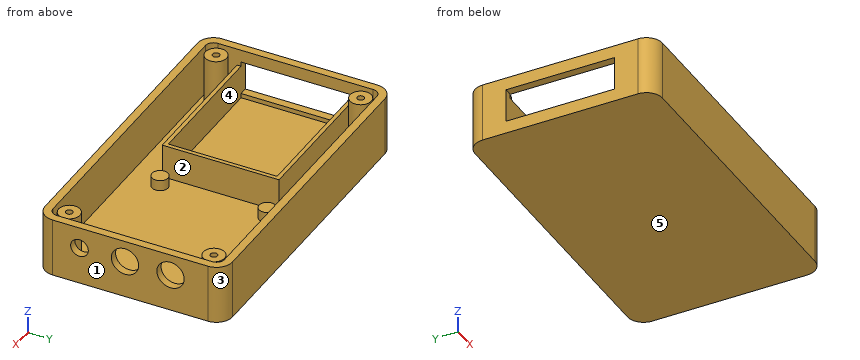
```python
from build123d import *

# Parameters (mm, degrees)
SKETCH1_W           = 120
SKETCH1_H           = 70
BOSS_EXTRUDE1_DEPTH = 22
FILLET1_R           = 6
SHELL1_T            = -3
SKETCH2_R           = 4
BOSS_EXTRUDE2_DEPTH = 18.0000001
SKETCH4_R           = 1.3
CUT_EXTRUDE1_DEPTH  = 4
BOSS_EXTRUDE3_DEPTH = 12.6
CUT_EXTRUDE2_REACH  = 128.921
SKETCH6_W           = 12.6
SKETCH6_H           = 40.6
CUT_EXTRUDE3_REACH  = 128.921
SKETCH8_R           = 5.1
SKETCH8_R_2         = 3.3
SKETCH9_R           = 3
BOSS_EXTRUDE4_DEPTH = 4


with BuildPart() as part:
    # Sketch1 → Boss-Extrude1 (new body)
    with BuildSketch(Plane.XY):
        Rectangle(SKETCH1_W, SKETCH1_H)
    extrude(amount=BOSS_EXTRUDE1_DEPTH)

    # Fillet1
    fillet1_edges = [part.edges().sort_by_distance(p)[0] for p in [
        (-60, 35, 11),
        (60, 35, 11),
        (60, -35, 11),
        (-60, -35, 11),
    ]]
    fillet(fillet1_edges, radius=FILLET1_R)

    # Shell1
    shell1_openings = [part.faces().sort_by_distance(p)[0] for p in [
        (0, 0, 22),
    ]]
    offset(amount=SHELL1_T, openings=shell1_openings, kind=Kind.INTERSECTION)

    # Sketch2 → Boss-Extrude2 (add)
    with BuildSketch(Plane.XY.offset(3)):
        with Locations((-52, -27)):
            Circle(SKETCH2_R)
        with Locations(Location((52, -27, 0), (0, 0, 180))):
            Circle(SKETCH2_R)
        with Locations((52, 27)):
            Circle(SKETCH2_R)
        with Locations(Location((-52, 27, 0), (0, 0, 180))):
            Circle(SKETCH2_R)
    extrude(amount=BOSS_EXTRUDE2_DEPTH)

    # Sketch4 → Cut-Extrude1 (cut)
    with BuildSketch(Plane.XY.offset(21.0000001)):
        with Locations((-52, 27)):
            Circle(SKETCH4_R)
        with Locations(Location((-52, -27, 0), (0, 0, 180))):
            Circle(SKETCH4_R)
        with Locations((52, -27)):
            Circle(SKETCH4_R)
        with Locations(Location((52, 27, 0), (0, 0, 180))):
            Circle(SKETCH4_R)
    extrude(amount=-CUT_EXTRUDE1_DEPTH, mode=Mode.SUBTRACT)

    # Sketch5 → Boss-Extrude3 (add)
    with BuildSketch(Plane(origin=(0, 0, 3), x_dir=(-1, 0, 0), z_dir=(0, 0, -1))):
        Polygon((57, 21.8), (4, 21.8), (4, -21.8), (57, -21.8), (57, -20.3), (5.5, -20.3), (5.5, 20.3), (57, 20.3), align=None)
    extrude(amount=-BOSS_EXTRUDE3_DEPTH)

    # Sketch6 → Cut-Extrude2 (cut, up to next)
    with BuildSketch(Plane(origin=(-60, 0, 0), x_dir=(0, 0, -1), z_dir=(1, 0, 0)), mode=Mode.PRIVATE) as cut_extrude2_sk1:
        with Locations((-11, 0)):
            Rectangle(SKETCH6_W, SKETCH6_H)
    cut_extrude2_tool1 = extrude(cut_extrude2_sk1.sketch, amount=CUT_EXTRUDE2_REACH, mode=Mode.PRIVATE) & part.part
    add(cut_extrude2_tool1.solids().sort_by_distance((-60, 0, 11))[0], mode=Mode.SUBTRACT)

    # Sketch8 → Cut-Extrude3 (cut, up to next)
    with BuildSketch(Plane.ZY.offset(-60), mode=Mode.PRIVATE) as cut_extrude3_sk1:
        with Locations(Location((14, 15, 0), (0, 0, 270))):
            Circle(SKETCH8_R)
    cut_extrude3_tool1 = extrude(cut_extrude3_sk1.sketch, amount=CUT_EXTRUDE3_REACH, mode=Mode.PRIVATE) & part.part
    # Sketch8 → Cut-Extrude3 (cut, up to next)
    with BuildSketch(Plane.ZY.offset(-60), mode=Mode.PRIVATE) as cut_extrude3_sk2:
        with Locations(Location((14, -2, 0), (0, 0, 270))):
            Circle(SKETCH8_R)
    cut_extrude3_tool2 = extrude(cut_extrude3_sk2.sketch, amount=CUT_EXTRUDE3_REACH, mode=Mode.PRIVATE) & part.part
    # Sketch8 → Cut-Extrude3 (cut, up to next)
    with BuildSketch(Plane.ZY.offset(-60), mode=Mode.PRIVATE) as cut_extrude3_sk3:
        with Locations(Location((14, -19, 0), (0, 0, 270))):
            Circle(SKETCH8_R_2)
    cut_extrude3_tool3 = extrude(cut_extrude3_sk3.sketch, amount=CUT_EXTRUDE3_REACH, mode=Mode.PRIVATE) & part.part
    add(cut_extrude3_tool1.solids().sort_by_distance((60, 15, 14))[0], mode=Mode.SUBTRACT)
    add(cut_extrude3_tool2.solids().sort_by_distance((60, -2, 14))[0], mode=Mode.SUBTRACT)
    add(cut_extrude3_tool3.solids().sort_by_distance((60, -19, 14))[0], mode=Mode.SUBTRACT)

    # Sketch9 → Boss-Extrude4 (add)
    with BuildSketch(Plane.XY.offset(3)):
        with Locations((43, 20)):
            Circle(SKETCH9_R)
        with Locations((1, 20)):
            Circle(SKETCH9_R)
        with Locations(Location((1, -20, 0), (0, 0, 180))):
            Circle(SKETCH9_R)
        with Locations(Location((43, -20, 0), (0, 0, 180))):
            Circle(SKETCH9_R)
    extrude(amount=BOSS_EXTRUDE4_DEPTH)


solid = part.part
```
Work out the finished part from the listing and answer in its coordinate system (mm). Face numbers are marked on the shaded views. A direction names the side the tool comes from. Round coordinates to 2 decimals unless told otherwise and drop trailing zeros. Write each loop counter-clockwise with the first axis right and the second up, starting at its lowest first coordinate (ties: lowest second). Pieces come first, ordered by that corner, then holes.
1) A cutting plane is placed at A-A on y = 15. Determine the outline of the cut face in (x, z), and give its area (4 significant figures).
2) Determine the mould class of the marked faces 3, 4 and 5 for opening direction Y: pulls with the +Y half, pulls with the -Y half, needs draft (parallel to the pull), parting line crosses it, or undercut.
3) A cutting plane is placed at D-D on x = -38.5. Determine the outline of the cut face in (y, z), and give its area (3 significant figures).
4) Flat-ended cylindrical pins translate along their axes: P1, Ø4, axis at y = -1, z = 8.5, coming from the -X side; P2, Ø2.5, axis at x = 52.5, y = 26.5, coming from the +Z side; P3, Ø1, axis at x = -23, y = -8, coming from the +Z side. Find the tip coordinate at first contact, or state that the pin passes through.
5) A cutting plane is placed at B-B on x = 1. Determine the outline of the cut face in (y, z), and give its area (3 significant figures).
6) A cutting plane is placed at C-C on y = 27. Determine the outline of the cut face in (x, z).
7) Which of the six approach directions +Z, -Z, +X, -X, +Y, -Y give full straight-line access (tool end or side, diameter ignored) to the marked faces 1 and 2?
8) Consider probe 1 along Y at (x, z) = (52, 18); probe 2 along Y at (x, z) = (-35, 6); probe 3 along Y at (x, z) = (-30, 17). Determine where each line is inside the solid, lowest interval first.
Entries:
1. outline: (-60, 0) - (60, 0) - (60, 8.9) - (57, 8.9) - (57, 3) - (-4, 3) - (-4, 15.6) - (-5.5, 15.6) - (-5.5, 3) - (-57, 3) - (-57, 4.7) - (-60, 4.7) - close; (-60, 17.3) - (-57, 17.3) - (-57, 22) - (-60, 22) - close; (57, 19.1) - (60, 19.1) - (60, 22) - (57, 22) - close
1. area: 424.5 mm2
2. face 3: pulls with the +Y half
2. face 4: undercut
2. face 5: needs draft
3. outline: (-35, 0) - (35, 0) - (35, 22) - (32, 22) - (32, 3) - (21.8, 3) - (21.8, 15.6) - (20.3, 15.6) - (20.3, 3) - (-20.3, 3) - (-20.3, 15.6) - (-21.8, 15.6) - (-21.8, 3) - (-32, 3) - (-32, 22) - (-35, 22) - close
3. area: 362 mm2
4. P1: stops at x = -5.5
4. P2: stops at z = 21
4. P3: stops at z = 3
5. outline: (-35, 0) - (35, 0) - (35, 22) - (32, 22) - (32, 3) - (23, 3) - (23, 7) - (17, 7) - (17, 3) - (-17, 3) - (-17, 7) - (-23, 7) - (-23, 3) - (-32, 3) - (-32, 22) - (-35, 22) - close
5. area: 372 mm2
6. outline: (-60, 0) - (60, 0) - (60, 22) - (57, 22) - (57, 3) - (56, 3) - (56, 21) - (53.3, 21) - (53.3, 17) - (50.7, 17) - (50.7, 21) - (48, 21) - (48, 3) - (-48, 3) - (-48, 21) - (-50.7, 21) - (-50.7, 17) - (-53.3, 17) - (-53.3, 21) - (-56, 21) - (-56, 3) - (-57, 3) - (-57, 22) - (-60, 22) - close
7. face 1: +Z, -Z, +X, +Y, -Y
7. face 2: +Z
8. probe 1: y = -35 to -32, -31 to -28.3, -25.7 to -23, 23 to 25.7, 28.3 to 31, 32 to 35
8. probe 2: y = -35 to -32, -21.8 to -20.3, 20.3 to 21.8, 32 to 35
8. probe 3: y = -35 to -32, 32 to 35
